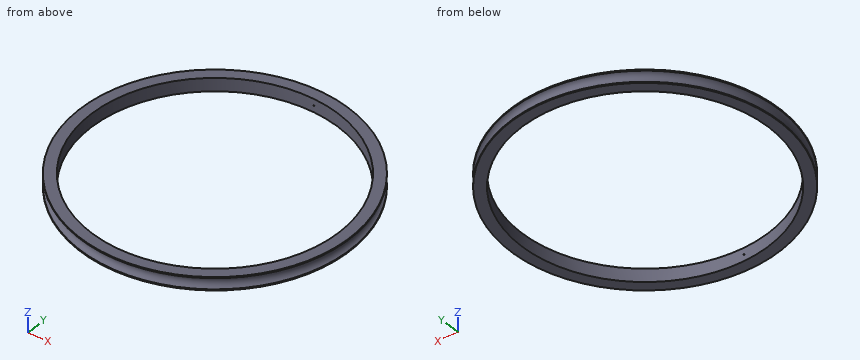
```python
from build123d import *

# Parameters (mm, degrees)
SKETCH3_R          = 0.5
CUT_EXTRUDE1_DEPTH = 29
SKETCH4_R          = 0.5
CUT_EXTRUDE2_DEPTH = 11


with BuildPart() as part:
    # Sketch1 → Revolve1 (revolve)
    with BuildSketch(Plane(origin=(0, 0, 0), x_dir=(0, 0, -1), z_dir=(1, 0, 0))):
        with BuildLine():
            Line((0.5, 113.24716621), (6, 113.24716621))
            Line((6, 113.24716621), (6, 123.24716621))
            Line((6, 123.24716621), (5, 123.24716621))
            ThreePointArc((5, 123.24716621), (0, 119.24716621), (-5, 123.24716621))
            Line((-5, 123.24716621), (-6, 123.24716621))
            Line((-6, 123.24716621), (-6, 113.24716621))
            Line((-6, 113.24716621), (-0.5, 113.24716621))
            Line((-0.5, 113.24716621), (0.5, 113.24716621))
        make_face()
    revolve(axis=Axis((0, 0, 80.785821763), (0, 0, -1)))

    # Sketch3 → Cut-Extrude1 (cut)
    with BuildSketch(Plane(origin=(0, 115.24716621, 0), x_dir=(-1, 0, 0), z_dir=(0, -1, 0))):
        Circle(SKETCH3_R)
    extrude(amount=CUT_EXTRUDE1_DEPTH, mode=Mode.SUBTRACT)

    # Sketch4 → Cut-Extrude2 (cut)
    with BuildSketch(Plane(origin=(0, -115.24716621, 0), x_dir=(1, 0, 0), z_dir=(0, 1, 0))):
        Circle(SKETCH4_R)
    extrude(amount=CUT_EXTRUDE2_DEPTH, mode=Mode.SUBTRACT)


solid = part.part
```
Check sheet for the modelled part. Datum: model origin and axes. Units: mm. Give positions to 0.01 mm unless a question says otherwise; leave off trailing zeros. Write each loop counter-clockwise with the first axis right and the second up, starting at its lowest first coordinate (ties: lowest second). Pieces come first, ordered by that corner, then holes.
Item 1: Cross-section at A-A (y = 0). Enter the section's corners in (x, z) (3 decimals).
Item 2: Scan lines: L1, parallel to Z at x = 0, y = 114; L2, parallel to X at y = 18, z = 2.5; L3, parallel to Y at x = -90, z = 4.25. Record each from-to range of solid material in increasing order.
Item 3: Gauge pin test, flat ends, axial feed: pin 1 (4 mm diameter, centred on y = 57, z = 0.5, fed in from +X); pin 2 (2 mm diameter, centred on y = -40.5, z = 0, fed in from +X); pin 3 (6 mm diameter, centred on x = -89, z = -3.5, fed in from -Y). Record the tip position at first contact, or that the pin passes through.
Item 4: Cross-section at B-B (z = -2.75). Enter the section's corners in (x, y), and give its area (3 significant figures).
Report:
1. outline: (-123.247, -6) - (-113.247, -6) - (-113.247, 6) - (-123.247, 6) - (-123.247, 5) arc R5.125 cw to (-123.247, -5) - close; (113.247, -6) - (123.247, -6) - (123.247, -5) arc R5.125 cw to (123.247, 5) - (123.247, 6) - (113.247, 6) - close
2. L1: z = -6 to -0.5, 0.5 to 6
2. L2: x = -118.54 to -111.81, 111.81 to 118.54
2. L3: y = -81.63 to -68.74, 68.74 to 81.63
3. pin 1: stops at x = 105.92
3. pin 2: stops at x = 112.52
3. pin 3: stops at y = -87.89
4. outline: circle Ø240.09 at (0, 0); hole circle Ø226.49 at (0, 0)
4. area: 4,980 mm2
